Work out the finished part from the listing and answer in its coordinate system (mm). Face numbers are marked on the shaded views. Give positions to 0.01 mm unless a question says otherwise; leave off trailing zeros. Order: outer loops, then holes, each group sorted by start corner. A loop starts at its lowest first (then second) coordinate and runs counter-clockwise, first axis right, second up. Notation, with made-up numbers: (2, 80) - (11, 80) arc R31 ccw to (11, 117) - close; hole circle Ø4 at (75, 47.25). An arc over 180 degrees is marked (long way). Return JSON: item names as keys, results as strings. Group by question number.
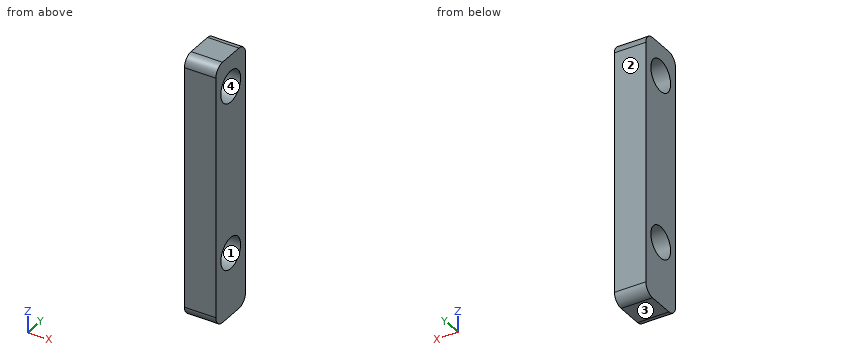
from build123d import *

# Parameters (mm, degrees)
SALIENTE_EXTRUIR1_DEPTH    = 1.5
CORTAR_EXTRUIR1_DEPTH      = 13.789155562
CORTAR_EXTRUIR1_DEPTH_BACK = 13.789155562
CROQUIS2_R                 = 1.5


with BuildPart() as part:
    # Croquis1 → Saliente-Extruir1 (new, symmetric)
    with BuildSketch(Plane(origin=(0, 0, 0), x_dir=(0, 0, -1), z_dir=(1, 0, 0))):
        with BuildLine():
            Line((-11.5, 2.25), (11.5, 2.25))
            ThreePointArc((11.5, 2.25), (12.207106781, 1.957106781), (12.5, 1.25))
            Line((12.5, 1.25), (12.5, -1.25))
            ThreePointArc((12.5, -1.25), (12.207106781, -1.957106781), (11.5, -2.25))
            Line((11.5, -2.25), (-11.5, -2.25))
            ThreePointArc((-11.5, -2.25), (-12.207106781, -1.957106781), (-12.5, -1.25))
            Line((-12.5, -1.25), (-12.5, 1.25))
            ThreePointArc((-12.5, 1.25), (-12.207106781, 1.957106781), (-11.5, 2.25))
        make_face()
    extrude(amount=SALIENTE_EXTRUIR1_DEPTH, both=True)

    # Croquis2 → Cortar-Extruir1 (cut, two sides: drawn at the far end of the back side and taken through both)
    with BuildSketch(Plane(origin=(0, 0, 0), x_dir=(0, 0, -1), z_dir=(1, 0, 0)).offset(-CORTAR_EXTRUIR1_DEPTH_BACK)):
        with Locations((-9.5, 0)):
            Circle(CROQUIS2_R)
        with Locations((6.5, 0)):
            Circle(CROQUIS2_R)
    extrude(amount=CORTAR_EXTRUIR1_DEPTH + CORTAR_EXTRUIR1_DEPTH_BACK, mode=Mode.SUBTRACT)


solid = part.part
1. Consider probe 1 along Z at (x, y) = (1.3, 0); probe 2 along Y at (x, z) = (0, 9.5); probe 3 along Z at (x, y) = (1.15, -0.9). Determine where each line is inside the solid, lowest interval first. Write a range as from..to.
2. The part is cut by section C-C (x = -0.9). Give the vertices of the cut face in (y, z), and give its area (3 significant figures).
3. This flat-tipped pin is pushed along its axis until it touches: pin 1 (1.8 mm diameter, centred on y = 0, z = 9.5, fed in from -X). Where does it stop, or does it pass through?
4. The part is cut by section B-B (y = 0). Give the vertices of the cut face in (x, z), and give its area (3 significant figures).
5. The part is cut by section A-A (z = 9.5). Give the vertices of the cut face in (x, y), and give its area (3 significant figures).
6. Determine the mould class of the marked faces 1, 2, 3 and 4 for opening direction Z: released by +Z, released by -Z, zero draft, split by the parting line, or undercut.
Answers:
{
 "1": {"probe 1": "z = -12.5..-8, -5..8, 11..12.5", "probe 2": "y = -2.25..-1.5, 1.5..2.25", "probe 3": "z = -12.5..-7.7, -5.3..8.3, 10.7..12.5"},
 "2": {"outline": "(-2.25, -11.5) arc R1 ccw to (-1.25, -12.5) - (1.25, -12.5) arc R1 ccw to (2.25, -11.5) - (2.25, 11.5) arc R1 ccw to (1.25, 12.5) - (-1.25, 12.5) arc R1 ccw to (-2.25, 11.5) - close; hole circle Ø3 at (0, -6.5); hole circle Ø3 at (0, 9.5)", "area": "97.5 mm^2"},
 "3": {"pin 1": "passes through"},
 "4": {"outline": "(-1.5, -12.5) - (1.5, -12.5) - (1.5, -8) - (-1.5, -8) - close; (-1.5, -5) - (1.5, -5) - (1.5, 8) - (-1.5, 8) - close; (-1.5, 11) - (1.5, 11) - (1.5, 12.5) - (-1.5, 12.5) - close", "area": "57.0 mm^2"},
 "5": {"outline": "(-1.5, -2.25) - (1.5, -2.25) - (1.5, -1.5) - (-1.5, -1.5) - close; (-1.5, 1.5) - (1.5, 1.5) - (1.5, 2.25) - (-1.5, 2.25) - close", "area": "4.50 mm^2"},
 "6": {"face 1": "undercut", "face 2": "zero draft", "face 3": "released by -Z", "face 4": "undercut"}
}
